from build123d import *

# Parameters (mm, degrees)
SKETCH1_W               = 18.5
SKETCH1_H               = 13
BOSS_EXTRUDE1_DEPTH     = 6
CUT_EXTRUDE1_DEPTH      = 21.506096654
CUT_EXTRUDE1_DEPTH_BACK = 21.506096654
SKETCH2_R               = 0.85
FILLET1_R               = 0.5
CHAMFER1_SIZE           = 5
CHAMFER2_SIZE           = 1.5


with BuildPart() as part:
    # Sketch1 → Boss-Extrude1 (new body)
    with BuildSketch(Plane(origin=(0, 0, 0), x_dir=(1, 0, 0), z_dir=(0, 1, 0))):
        with Locations((9.25, 0)):
            Rectangle(SKETCH1_W, SKETCH1_H)
    extrude(amount=BOSS_EXTRUDE1_DEPTH)

    # Sketch2 → Cut-Extrude1 (cut, two sides: drawn at the far end of the back side and taken through both)
    with BuildSketch(Plane(origin=(0, 6, 0), x_dir=(1, 0, 0), z_dir=(0, 1, 0)).offset(-CUT_EXTRUDE1_DEPTH_BACK)):
        with Locations(Location((2.5, 3.25, 0), (0, 0, 270))):
            Circle(SKETCH2_R)
        with Locations(Location((2.5, -3.25, 0), (0, 0, 270))):
            Circle(SKETCH2_R)
    extrude(amount=CUT_EXTRUDE1_DEPTH + CUT_EXTRUDE1_DEPTH_BACK, mode=Mode.SUBTRACT)

    # Fillet1
    fillet1_edges = [part.edges().sort_by_distance(p)[0] for p in [
        (2.5, 0, -4.1),
        (2.5, 6, -4.1),
        (2.5, 0, 2.4),
        (2.5, 6, 2.4),
    ]]
    fillet(fillet1_edges, radius=FILLET1_R)

    # Chamfer1
    chamfer1_edges = [part.edges().sort_by_distance(p)[0] for p in [
        (18.5, 3, 6.5),
    ]]
    chamfer(chamfer1_edges, length=CHAMFER1_SIZE)

    # Chamfer2
    chamfer2_edges = [part.edges().sort_by_distance(p)[0] for p in [
        (18.5, 0, -2.5),
        (18.5, 6, -2.5),
        (16, 0, 4),
        (16, 6, 4),
    ]]
    chamfer(chamfer2_edges, length=CHAMFER2_SIZE)


solid = part.part
Part model, mm, in its own coordinate system. Coordinates: 2 decimals unless noted, no trailing zeros. Loops run counter-clockwise (first coordinate to the right, second up) from the corner with the lowest first, then second, coordinate; pieces in that order, holes last. Notation, with made-up numbers: M 89,55 L 146,55 A16 cw 146,77 Z; hole C 78,71.25 d8. An arc over 180 degrees is marked long. Use a Markdown table: item, result. Add a question column.
Q1. Cut at B-B (y = 2.25). Write the cut outline in (x, z), and give its area (3 significant figures).
Q2. Cut at C-C (x = 2.5). Write the cut outline in (y, z).
Q3. Pin check, flat tips, straight feed: P1, Ø2.5, axis at x = 2.5, z = 3.25, coming from the +Y side; P2, Ø2, axis at x = 2.5, z = -3.25, coming from the -Y side. Stop position of each tip, or through.
Q4. Cut at A-A (z = -3.25). Write the cut outline in (x, y).
Q5. Probe L1, parallel to Z at x = 2.5, y = 2.05; L2, parallel to X at y = 2, z = -3.25; L3, parallel to Z at x = 3, y = 5. List the from-to ranges inside material, lowest first.
Q6. Cut at D-D (z = 3.25). Write the cut outline in (x, y).
Worked out:
| question | item | result |
|---|---|---|
| 1 | outline | M 0,-6.5 L 18.5,-6.5 L 18.5,1.5 L 13.5,6.5 L 0,6.5 Z; hole C 2.5,-3.25 d1.7; hole C 2.5,3.25 d1.7 |
| 1 | area | 223 mm2 |
| 2 | outline | M 0,-6.5 L 6,-6.5 L 6,-4.6 A0.5 ccw 5.5,-4.1 L 0.5,-4.1 A0.5 ccw 0,-4.6 Z; M 0,-1.9 A0.5 ccw 0.5,-2.4 L 5.5,-2.4 A0.5 ccw 6,-1.9 L 6,1.9 A0.5 ccw 5.5,2.4 L 0.5,2.4 A0.5 ccw 0,1.9 Z; M 0,4.6 A0.5 ccw 0.5,4.1 L 5.5,4.1 A0.5 ccw 6,4.6 L 6,6.5 L 0,6.5 Z |
| 3 | P1 | stops at y = 5.99 |
| 3 | P2 | stops at y = 0.14 |
| 4 | outline | M 0,0 L 1.15,0 A0.5 ccw 1.65,0.5 L 1.65,5.5 A0.5 ccw 1.15,6 L 0,6 Z; M 3.35,0.5 A0.5 ccw 3.85,0 L 17,0 L 18.5,1.5 L 18.5,4.5 L 17,6 L 3.85,6 A0.5 ccw 3.35,5.5 Z |
| 5 | L1 | z = -6.5 to -4.1, -2.4 to 2.4, 4.1 to 6.5 |
| 5 | L2 | x = 0 to 1.65, 3.35 to 18.5 |
| 5 | L3 | z = -6.5 to -3.94, -2.56 to 2.56, 3.94 to 6.5 |
| 6 | outline | M 0,0 L 1.15,0 A0.5 ccw 1.65,0.5 L 1.65,5.5 A0.5 ccw 1.15,6 L 0,6 Z; M 3.35,0.5 A0.5 ccw 3.85,0 L 14.63,0 L 16.75,1.5 L 16.75,4.5 L 14.63,6 L 3.85,6 A0.5 ccw 3.35,5.5 Z |
